```python
from build123d import *

# Parameters (mm, degrees)
SKETCH1_W           = 75
SKETCH1_H           = 168
BOSS_EXTRUDE1_DEPTH = 3
SKETCH2_R           = 1
CUT_EXTRUDE1_DEPTH  = 93.03939374
SKETCH3_W           = 10
SKETCH3_H           = 10
BOSS_EXTRUDE2_DEPTH = 3


with BuildPart() as part:
    # Sketch1 → Boss-Extrude1 (new body)
    with BuildSketch(Plane.XY):
        Rectangle(SKETCH1_W, SKETCH1_H)
    extrude(amount=BOSS_EXTRUDE1_DEPTH)

    # Sketch2 → Cut-Extrude1 (cut, through all)
    with BuildSketch(Plane.XY.offset(3)):
        with Locations((36, 82.5)):
            Circle(SKETCH2_R)
        with Locations(Location((-36, 82.5, 0), (0, 0, 180))):
            Circle(SKETCH2_R)
        with Locations(Location((36, -82.5, 0), (0, 0, 180))):
            Circle(SKETCH2_R)
        with Locations((-36, -82.5)):
            Circle(SKETCH2_R)
    extrude(amount=-CUT_EXTRUDE1_DEPTH, mode=Mode.SUBTRACT)

    # Sketch3 → Boss-Extrude2 (add)
    with BuildSketch(Plane.XY.offset(3)):
        with Locations((42.5, 0)):
            Rectangle(SKETCH3_W, SKETCH3_H)
    extrude(amount=-BOSS_EXTRUDE2_DEPTH)


solid = part.part
```
Could you check a few things on this model? Use its own coordinates, in mm. A direction names the side the tool comes from. Coordinates: 2 decimals unless noted, no trailing zeros. Loops run counter-clockwise (first coordinate to the right, second up) from the corner with the lowest first, then second, coordinate; pieces in that order, holes last.
1) Please list where these lines run through material, in increasing order: line 1 along X through (y, z) = (82.5, 1.85); line 2 along Y through (x, z) = (-36, 1.8); line 3 along X through (y, z) = (38, 0.8).
Reported:
line 1: x = -37.5 to -37, -35 to 35, 37 to 37.5
line 2: y = -84 to -83.5, -81.5 to 81.5, 83.5 to 84
line 3: x = -37.5 to 37.5
2) Imagine slicing it at A-A (z = 0.9). List the corners of the cut face in (x, y) for me.
Reported:
outline: (-37.5, -84) - (37.5, -84) - (37.5, -5) - (47.5, -5) - (47.5, 5) - (37.5, 5) - (37.5, 84) - (-37.5, 84) - close; hole circle Ø2 at (-36, -82.5); hole circle Ø2 at (-36, 82.5); hole circle Ø2 at (36, -82.5); hole circle Ø2 at (36, 82.5)
3) Thinking about a two-plate mould opening in Z: for faces 4 (the face through (-37.5, -1, 1)), 5 (the face through (4, 1, 0)), 6 (the face through (4, 1, 3)), which applies, released by +Z, released by -Z, zero draft, split by the parting line, or undercut?
Reported:
face 4: zero draft
face 5: released by -Z
face 6: released by +Z
4) Will these pins go through, and if not, where does the flat tip stop? pin 1 Ø1.8 at (x, y) = (36, -82.5) entering from -Z; pin 2 Ø0.9 at (x, z) = (41, 1.5) entering from -Y; pin 3 Ø0.9 at (y, z) = (63, 2) entering from +X.
Reported:
pin 1: passes through
pin 2: stops at y = -5
pin 3: stops at x = 37.5
5) Which directions (+Z, -Z, +X, -X, +Y, -Y) give clear straight access to the entire face, cutting with the end or side of a thin tool? Please do faces 1 (the face through (-1, 84, 1)), 2 (the face through (42, -5, 2)), 3 (the face through (42, 5, 2)).
Reported:
face 1: +Z, -Z, +X, -X, +Y
face 2: +Z, -Z, +X, -Y
face 3: +Z, -Z, +X, +Y
6) Imagine slicing it at B-B (y = -11). List the corners of the cut face in (x, z) for me, and give its area (3 significant figures).
Reported:
outline: (-37.5, 0) - (37.5, 0) - (37.5, 3) - (-37.5, 3) - close
area: 225 mm2
